from build123d import *

# Parameters (mm, degrees)
F0_W     = 228.6
F0_H     = 177.8
F1_DEPTH = 23.8125
F2_R     = 72.445
F3_DEPTH = 25.4
F2_R_2   = 85.5
F4_DEPTH = 6.5
F5_R     = 12.7
F6_R     = 12.7
F7_SIZE  = 12.7


with BuildPart() as f1:
    # F0 (on Front) → F1 (new body)
    with BuildSketch(Plane.XZ):
        with Locations((-38.534197, -24.81398)):
            Rectangle(F0_W, F0_H)
    extrude(amount=F1_DEPTH)

    # F2 (on face) → F3 (cut)
    with BuildSketch(Plane.XZ.offset(23.8125)):
        with Locations((-38.534197, -24.81398)):
            Circle(F2_R)
    extrude(amount=-F3_DEPTH, mode=Mode.SUBTRACT)

    # F2 (on face) → F4 (cut)
    with BuildSketch(Plane.XZ.offset(23.8125)):
        with Locations((-38.534197, -24.81398)):
            Circle(F2_R_2)
        with Locations((-38.534197, -24.81398)):
            Circle(F2_R, mode=Mode.SUBTRACT)
    extrude(amount=-F4_DEPTH, mode=Mode.SUBTRACT)

    # F5
    f5_edges = [f1.edges().sort_by_distance(p)[0] for p in [
        (75.765803, -23.8125, -24.81398),
    ]]
    fillet(f5_edges, radius=F5_R)

    # F6
    f6_edges = [f1.edges().sort_by_distance(p)[0] for p in [
        (-152.834197, -23.8125, -24.81398),
    ]]
    fillet(f6_edges, radius=F6_R)

    # F7
    f7_edges = [f1.edges().sort_by_distance(p)[0] for p in [
        (-110.979197, 0, -24.81398),
    ]]
    chamfer(f7_edges, length=F7_SIZE)


solid = f1.part
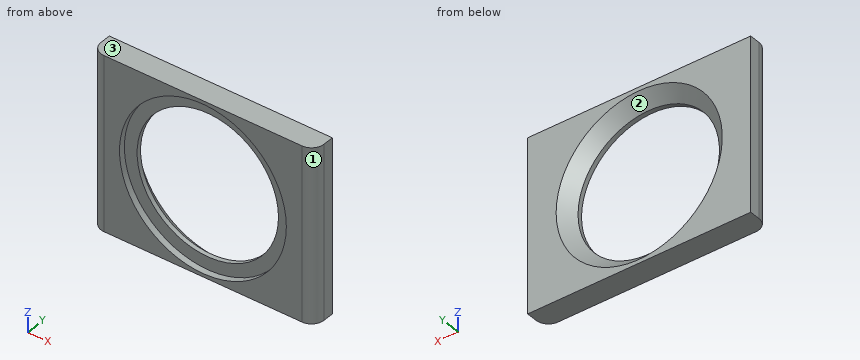
The listing builds one solid part. Answer for the finished solid, in the listing's coordinates (mm). Face numbers are marked on the shaded views. Give positions to 0.01 mm unless a question says otherwise; leave off trailing zeros. Write each loop counter-clockwise with the first axis right and the second up, starting at its lowest first coordinate (ties: lowest second). Pieces come first, ordered by that corner, then holes.
Item 1: Determine the mould class of the marked faces 1, 2 and 3 for opening direction X: released by +X, released by -X, zero draft, split by the parting line, or undercut.
Item 2: Find the intervals of material crossed by line 1 along Z through (x, y) = (36, -21); line 2 along Z through (x, y) = (26, -0.75); line 3 along X through (y, z) = (-7.5, -28), in increasing order.
Item 3: Section A-A, the plane y = -3.25 is taken. Write down the section's boundary in (x, z) (3 decimals), plus the area to 3 significant figures.
Item 4: Flat-ended cylindrical pins translate along their axes: P1, Ø6, axis at y = -13, z = -75, coming from the +X side; P2, Ø8, axis at y = -20.5, z = -34, coming from the -X side; P3, Ø2, axis at y = -18.5, z = 6, coming from the -X side. Find the tip coordinate at first contact, or state that the pin passes through.
Completed:
1. face 1: released by +X
1. face 2: undercut
1. face 3: zero draft
2. line 1: z = -113.71 to -66.71, 17.08 to 64.09
2. line 2: z = -113.71 to -79.2, 29.57 to 64.09
2. line 3: x = -152.83 to -116.11, 39.05 to 75.77
3. outline: (-152.834, -113.714) - (75.766, -113.714) - (75.766, 64.086) - (-152.834, 64.086) - close; hole circle Ø163.79 at (-38.534, -24.814)
3. area: 19,600 mm2
4. P1: stops at x = 75.77
4. P2: stops at x = -151.63
4. P3: stops at x = -151.11
